The drawing under review shows one solid part. Ordinate dimensions are in mm from its lowest x, y, z. A direction names the side the tool comes from. Coordinates: 2 decimals unless noted, no trailing zeros. Order: outer loops, then holes, each group sorted by start corner. A loop starts at its lowest first (then second) coordinate and runs counter-clockwise, first axis right, second up. Notation, with made-up numbers: (88, 83) -> (95, 83) arc R27 cw to (95, 111) -> close; hole circle Ø10 at (62.5, 67). An arc over 180 degrees is marked (long way). Use a Markdown table: item, result. Add a question column.
Q1. Add section D-D (x = 21.25). State the section outline as (y, z) points, then the cut area to 3 significant figures.
Q2. Add section C-C (y = 4). State the section outline as (x, z) points, then the cut area to 3 significant figures.
Q3. Add section A-A (x = 4). State the section outline as (y, z) points, then the cut area to 3 significant figures.
Q4. The part is to be moulded in two halves that separate along Y. For the marked faces 1, 2 and 3, say which applies: pulls with the +Y half, pulls with the -Y half, needs draft (parallel to the pull), parting line crosses it, or undercut.
Q5. Machinability: for the marked faces 4 and 5, which of the approach directions +Z, -Z, +X, -X, +Y, -Y give a long, thin tool a straight path to every point of the face, cutting with its end or side? Answer none if there is none.
Q6. Add section B-B (z = 1.6). State the section outline as (x, y) points.
Q7. Wall thickness on probe 1 along Y at (x, z) = (24, 2.55); probe 2 along Y at (x, z) = (4, 1.3); probe 3 along Y at (x, z) = (23.5, 4.3): over which ranges is each line inside the solid? List them lowest first.
Q8. Insertion check: pin 1 (2 mm diameter, centred on x = 24, y = 24, fed in from -Z); pin 2 (4.5 mm diameter, centred on x = 4, y = 24, fed in from +Z); pin 3 (3 mm diameter, centred on x = 24, y = 4, fed in from +Z). Each pin has a flat end and moves straight along its axis. Give the tip position at first contact, or say it passes through.
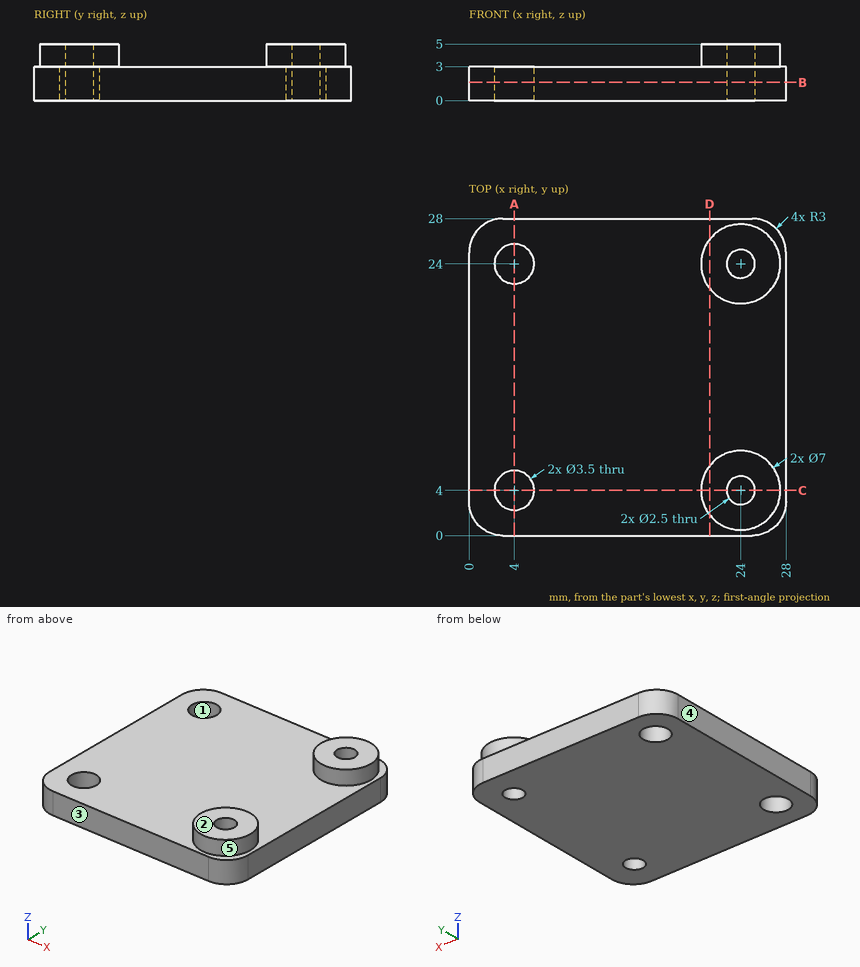
Established:
| question | item | result |
|---|---|---|
| 1 | outline | (0, 0) -> (28, 0) -> (28, 3) -> (26.17, 3) -> (26.17, 5) -> (21.83, 5) -> (21.83, 3) -> (6.17, 3) -> (6.17, 5) -> (1.83, 5) -> (1.83, 3) -> (0, 3) -> close |
| 1 | area | 101 mm^2 |
| 2 | outline | (0, 0) -> (2.25, 0) -> (2.25, 3) -> (0, 3) -> close; (5.75, 0) -> (22.75, 0) -> (22.75, 5) -> (20.5, 5) -> (20.5, 3) -> (5.75, 3) -> close; (25.25, 0) -> (28, 0) -> (28, 3) -> (27.5, 3) -> (27.5, 5) -> (25.25, 5) -> close |
| 2 | area | 75.0 mm^2 |
| 3 | outline | (0, 0) -> (2.25, 0) -> (2.25, 3) -> (0, 3) -> close; (5.75, 0) -> (22.25, 0) -> (22.25, 3) -> (5.75, 3) -> close; (25.75, 0) -> (28, 0) -> (28, 3) -> (25.75, 3) -> close |
| 3 | area | 63.0 mm^2 |
| 4 | face 1 | undercut |
| 4 | face 2 | needs draft |
| 4 | face 3 | pulls with the -Y half |
| 5 | face 4 | +Z, -Z, -X, +Y, -Y |
| 5 | face 5 | +Z |
| 6 | outline | (0, 3) arc R3 ccw to (3, 0) -> (25, 0) arc R3 ccw to (28, 3) -> (28, 25) arc R3 ccw to (25, 28) -> (3, 28) arc R3 ccw to (0, 25) -> close; hole circle Ø3.5 at (4, 4); hole circle Ø3.5 at (4, 24); hole circle Ø2.5 at (24, 4); hole circle Ø2.5 at (24, 24) |
| 7 | probe 1 | 0 to 2.75, 5.25 to 22.75, 25.25 to 28 |
| 7 | probe 2 | 0 to 2.25, 5.75 to 22.25, 25.75 to 28 |
| 7 | probe 3 | 0.54 to 2.85, 5.15 to 7.46, 20.54 to 22.85, 25.15 to 27.46 |
| 8 | pin 1 | through |
| 8 | pin 2 | z = 3 |
| 8 | pin 3 | z = 5 |
